Part print with two shaded views. Sizes in mm from the minimum x, y, z corner. Coordinates: 2 decimals unless noted, no trailing zeros. Order: outer loops, then holes, each group sorted by start corner. A loop starts at its lowest first (then second) coordinate and runs counter-clockwise, first axis right, second up. Notation, with made-up numbers: (-28, 78.25) - (-20, 78.25) arc R30 ccw to (-20, 101.25) - close; hole circle Ø1 at (67, 42.25). An arc over 180 degrees is marked (long way). One line per item, written item: value.
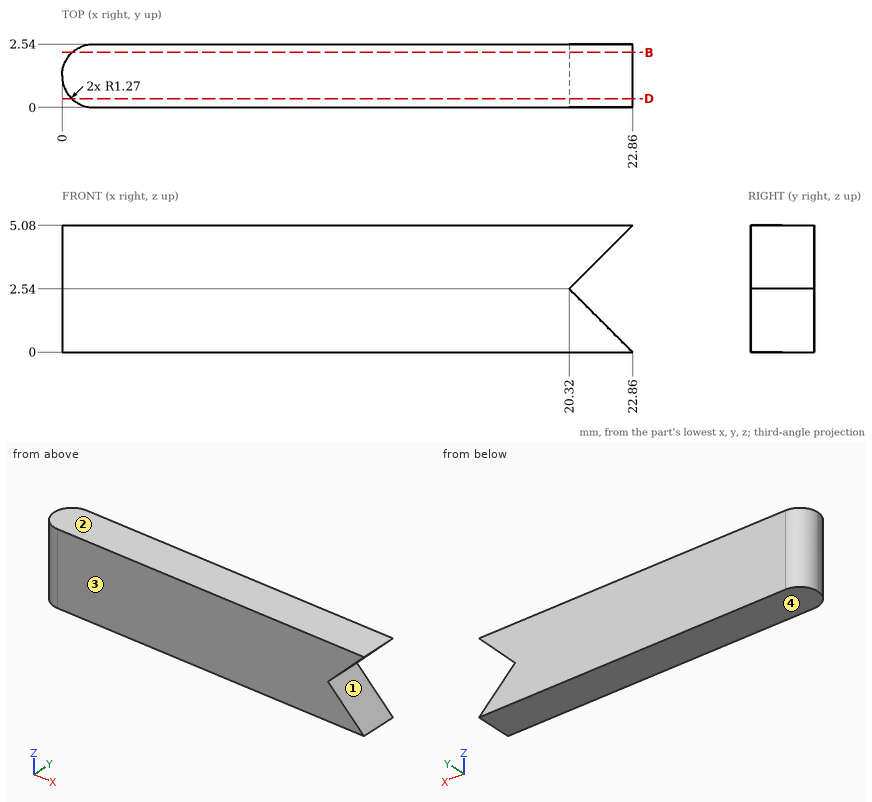
1. Two-plate mould, pull along Z, no slides. Class the marked faces 1, 2, 3 and 4: pulls with the +Z half, pulls with the -Z half, needs draft (parallel to the pull), parting line crosses it, or undercut.
Values found:
face 1: undercut
face 2: pulls with the +Z half
face 3: needs draft
face 4: pulls with the -Z half
2. Probe line 1 along X through (y, z) = (2.1, 4.5); line 2 along X through (y, z) = (0.7, 1.25) (1 decimal); line 3 along Y through (x, z) = (1, 3.7). List the from-to ranges inside material, lowest first.
Values found:
line 1: x = 0.31 to 22.28
line 2: x = 0.1 to 21.6
line 3: y = 0.03 to 2.51
3. Flat gauge pin, fed straight in: P1, Ø1.5, axis at y = 2, z = 3.5, coming from the -X side. Where does the tip first touch, or does it go through?
Values found:
P1: stops at x = 0
4. Band-saw the part on D-D, the plane y = 0.35. Give the cut face in (x, z).
Values found:
outline: (0.39, 0) - (22.86, 0) - (20.32, 2.54) - (22.86, 5.08) - (0.39, 5.08) - close
5. Band-saw the part on B-B, the plane y = 2.2. Give the cut face in (x, z) (3 decimals).
Values found:
outline: (0.405, 0) - (22.86, 0) - (20.32, 2.54) - (22.86, 5.08) - (0.405, 5.08) - close
